Input: part model. Units: mm. Frame: model coordinates. Face numbers are marked on the shaded views. A direction names the side the tool comes from. Coordinates: 2 decimals unless noted, no trailing zeros. Order: outer loops, then holes, each group sorted by start corner. A loop starts at its lowest first (then second) coordinate and runs counter-clockwise, first axis right, second up. Notation, with made-up numbers: (35.5, 20.25) -> (56.5, 20.25) arc R19 cw to (56.5, 54.25) -> close; hole circle Ø4 at (-22.75, 21). An arc over 180 degrees is marked (long way). Use one line per item in the form item = value. Start each with the question number.
1) Section query A-A on z = 0. Output: boundary loops of the cut face in (x, y).
2) Pin query (flat end, axial travel): pin 1 (2 mm diameter, centred on x = 4, y = 0.5, fed in from +Z); pin 2 (3 mm diameter, centred on y = 1, z = -5.5, fed in from +X); pin 3 (2 mm diameter, centred on x = 7.42, y = 0, fed in from +Z). Return the tip coordinate at first contact, or that it passes through.
3) Access query for the marked faces 1, 2 and 3. Directions: +Z, -Z, +X, -X, +Y, -Y. A direction counts if a zero-diameter tool reaches every point of the face in a straight line with its end or side. Return the directions, or none.
4) Section query D-D on y = 2.5. Output: boundary loops of the cut face in (x, z), then the cut area to 3 significant figures.
5) Ray query, line 1 along Z through (x, y) = (0, -0.5); line 2 along X through (y, z) = (0, 0.15); line 3 along X through (y, z) = (-2, 4). Return the intervals inside material, ascending.
6) Section query B-B on x = 0. Output: boundary loops of the cut face in (y, z).
7) Draft query along Y for the marked faces 4, 5 and 6. Return one class per face: pulls with the +Y half, pulls with the -Y half, needs draft (parallel to the pull), parting line crosses it, or undercut.
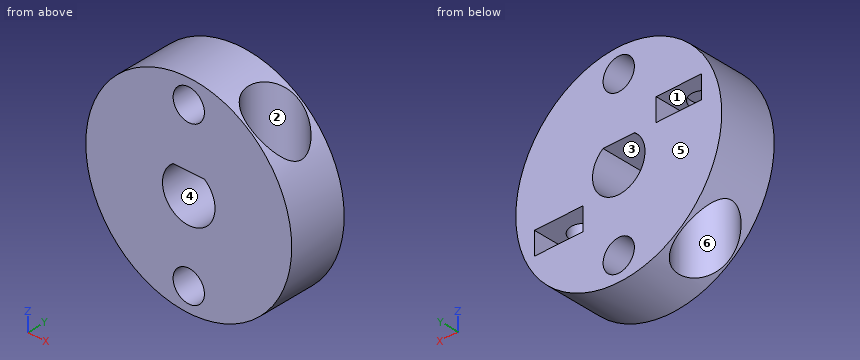
Autodesk Inventor part; units mm, degrees
ref_plane "Work Plane1" through (0, 0, 2.5) normal (0, 0, 1) x (1, 0, 0)
ref_plane "Work Plane2" through (0, 0, -2.5) normal (0, 0, 1) x (1, 0, 0)
ref_plane "Work Plane3" through (0, 5.3975, 0) normal (0, 1, 0) x (1, 0, 0)
sketch "Sketch1" plane through (0, 0, 0) normal (0, 1, 0) x (-1, 0, 0)
  circle A0 centre (0, 0) radius 12.7
  dimension "d75" = 25.4
extrude "Extrusion1" add sketch "Sketch1" along normal blind 3.4925 and the other way blind 3.4925
ref_plane "Work Plane1" through (0, 0, 2.5) normal (0, 0, 1) x (1, 0, 0)
ref_plane "Work Plane2" through (0, 0, -2.5) normal (0, 0, 1) x (1, 0, 0)
sketch "Sketch2" plane through (0, 0, 0) normal (0, 0, 1) x (1, 0, 0)
  circle A0 centre (7.4168, 0) radius 1.7
  circle A1 centre (-7.4168, 0) radius 1.7
  point P0 (0, 0)
  dimension "d5" = 3.4
  dimension "d6" = 7.4168
  dimension "d7" = 3.4
  dimension "d8" = 7.4168
extrude "Screw hole 2" cut sketch "Sketch2" along normal blind 2.5 and the other way blind 6 contours A0
sketch "Sketch3" plane through (0, 0, 2.5) normal (0, 0, 1) x (1, 0, 0)
  circle A0 centre (7.4168, 0) radius 1.7
  circle A1 centre (7.4168, 0) radius 3.25
  point P0 (0, 0)
  dimension "d19" = 6.5
sketch "Sketch4" plane through (0, 0, -2.5) normal (0, 0, 1) x (1, 0, 0)
  circle A0 centre (7.4168, 0) radius 1.7
  circle A1 centre (7.4168, 0) radius 3.45 construction
  line L0 (7.4168, -3.45) -> (4.429, -1.725)
  line L1 (4.429, -1.725) -> (4.429, 6.985)
  line L2 (10.4046, 6.985) -> (10.4046, -1.725)
  line L3 (10.4046, -1.725) -> (7.4168, -3.45)
  line L4 (10.4046, 6.985) -> (4.429, 6.985)
  point P0 (0, 0)
  dimension "d22" = 6.9
sketch "Sketch5" plane through (0, 0, -2.5) normal (0, 0, 1) x (1, 0, 0)
  circle A0 centre (-7.422, 0) radius 3.25
  point P0 (0, 0)
  dimension "d25" = 6.5
extrude "Access Hole 1" cut sketch "Sketch5" against normal through all
extrude "Access Hole 2" cut sketch "Sketch3" along normal through all contours A0 | A1
extrude "Nut well 2" cut sketch "Sketch4" against normal blind 2.794 contours A0 | L0 L1 L4 L2 L3
sketch "Sketch7" plane through (0, 0, 2.5) normal (0, 0, 1) x (1, 0, 0)
  circle A0 centre (-7.422, 0) radius 3.25 construction
  circle A1 centre (-7.422, 0) radius 3.45 construction
  line L0 (-7.422, -3.25) -> (-10.2365, -1.625)
  line L1 (-10.2365, -1.625) -> (-10.2365, 5.3975)
  line L2 (-4.6074, 5.3975) -> (-4.6074, -1.625)
  line L3 (-4.6074, -1.625) -> (-7.422, -3.25)
  line L4 (16.6201, 5.3975) -> (-16.6201, 5.3975)
  line L5 (-10.2365, 5.3975) -> (-4.6074, 5.3975)
  point P0 (0, 0)
  dimension "d48" = 6.9
extrude "Nut Well 1" cut sketch "Sketch7" along normal blind 2.794
sketch "Sketch8" plane through (0, 0, 0) normal (0, 0, 1) x (1, 0, 0)
  circle A0 centre (-7.422, 0) radius 3.25
  circle A1 centre (-7.422, 0) radius 1.7
  point P0 (0, 0)
  dimension "d51" = 3.4
extrude "Screw Hole 1" cut sketch "Sketch8" along normal blind 6 and the other way blind 2.5 contours A1
ref_plane "Work Plane3" through (0, 5.3975, 0) normal (0, 1, 0) x (1, 0, 0)
sketch "Sketch9" plane through (0, 5.3975, 0) normal (0, 1, 0) x (1, 0, 0)
  arc A0 (1.9431, -2.5908) -> (-1.9431, -2.5908) centre (0, 0) ccw
  line L0 (-1.9431, -2.5908) -> (1.9431, -2.5908)
  dimension "d56" = 6.477
  dimension "d57" = 2.5908
extrude "Center shaft" cut sketch "Sketch9" against normal through all
ref_plane "Work Plane4" through (0, 5.3975, 0) normal (0, 1, 0) x (1, 0, 0)
sketch "Sketch10" plane through (0, 5.3975, 0) normal (0, 1, 0) x (1, 0, 0)
  circle A0 centre (0, 9.779) radius 1.9304
  circle A1 centre (0, -9.779) radius 1.9304
  point P0 (0, 0)
  point P1 (0, -8.001)
  dimension "d60" = 3.8608
  dimension "d61" = 9.779
  dimension "d62" = 3.8608
  dimension "d63" = 9.779
extrude "Wheel holes" cut sketch "Sketch10" against normal through all
properties part number "clamping hub .770 .25 D bore base"
Answers below:
q1.outline = (-12.7, -3.49) -> (-3.24, -3.49) -> (-3.24, 3.49) -> (-12.7, 3.49) -> close; (3.24, -3.49) -> (12.7, -3.49) -> (12.7, 3.49) -> (3.24, 3.49) -> close; hole circle Ø3.4 at (-7.42, 0); hole circle Ø3.4 at (7.42, 0)
q2.pin_1 = 12.34
q2.pin_2 = 12.05
q2.pin_3 = -6
q3.face_1 = +Y
q3.face_2 = +Z
q3.face_3 = +Y, -Y
q4.outline = (-9.5, -8.43) -> (-9.5, -2.5) -> (-5.35, -2.5) -> (-5.35, -11.52) arc R12.7 ccw to (9.49, 8.44) -> (9.49, 2.5) -> (5.34, 2.5) -> (5.34, 11.52) arc R12.7 ccw to start; hole (-10.24, 2.5) -> (-4.61, 2.5) -> (-4.61, 5.29) -> (-10.24, 5.29) -> close; hole (-1.94, 2.59) arc R3.24 ccw (long way) to (1.94, 2.59) -> close; hole circle Ø3.86 at (0, -9.78); hole circle Ø3.86 at (0, 9.78); hole (4.43, -5.29) -> (10.4, -5.29) -> (10.4, -2.5) -> (4.43, -2.5) -> close
q4.area = 356 mm^2
q5.line_1 = -12.7 to -11.71, -7.85 to -3.24, 2.59 to 7.85, 11.71 to 12.7
q5.line_2 = -12.7 to -9.12, -5.72 to -3.24, 3.24 to 5.72, 9.12 to 12.7
q5.line_3 = -12.05 to -9.59, -5.26 to 4.86, 9.98 to 12.05
q6.outline = (-3.49, -12.7) -> (3.49, -12.7) -> (3.49, -11.71) -> (-3.49, -11.71) -> close; (-3.49, -7.85) -> (3.49, -7.85) -> (3.49, -3.24) -> (-3.49, -3.24) -> close; (-3.49, 2.59) -> (3.49, 2.59) -> (3.49, 7.85) -> (-3.49, 7.85) -> close; (-3.49, 11.71) -> (3.49, 11.71) -> (3.49, 12.7) -> (-3.49, 12.7) -> close
q7.face_4 = needs draft
q7.face_5 = pulls with the +Y half
q7.face_6 = undercut
